```python
from build123d import *

# Parameters (mm, degrees)
F0_R     = 9
F1_DEPTH = 8
F2_R     = 3
F3_SIZE  = 7.99999
F4_SIZE2 = 7.7942286341
F4_SIZE  = 4.5


# Not quite as in the source:
# - a fillet or chamfer is up to 0.001 mm smaller than in the source, because OpenCascade refuses the exact size
# - ends of sketch curves that miss each other by under 0.0002 mm in the source are joined


with BuildPart() as f1:
    # F0 (on Front) → F1 (new body)
    with BuildSketch(Plane.XZ):
        with BuildLine():
            ThreePointArc((-43, -330.994167), (0, -287.994167), (43, -330.994167))
            ThreePointArc((43, -330.994167), (109.276026714, -321.904147751), (174.0000001055, -304.9941673237))
            Line((174.0000001055, -304.9941673237), (167.462801, -276.227606))
            Line((167.462801, -276.227606), (105.54156, -290.299203))
            ThreePointArc((105.54156, -290.299203), (85.7953886494, -277.8658315797), (98.2287608958, -258.1196605414))
            Line((98.2287608958, -258.1196605414), (160.150002, -244.048063))
            Line((160.150002, -244.048063), (101.992538, 11.87045))
            Line((101.992538, 11.87045), (133.663965, 45.228522))
            Line((133.663965, 45.228522), (88.338787, 88.261977))
            ThreePointArc((88.338787, 88.261977), (87.7337722092, 111.5886563014), (111.0604515643, 112.1936705411))
            Line((111.0604515643, 112.1936705411), (156.385629, 69.160216))
            Line((156.385629, 69.160216), (187.038105, 101.445071))
            Line((187.038105, 101.445071), (191.402576, 146.180902))
            Line((191.402576, 146.180902), (129.197911, 152.24965))
            ThreePointArc((129.197911, 152.24965), (114.3780295485, 170.2738304953), (132.4022099517, 185.0937125046))
            Line((132.4022099517, 185.0937125046), (194.606875, 179.024965))
            Line((194.606875, 179.024965), (198.96141, 223.658948))
            Line((198.96141, 223.658948), (169.162302, 256.167065))
            Line((169.162302, 256.167065), (123.090168, 213.934276))
            ThreePointArc((123.090168, 213.934276), (99.7776684169, 214.9478629238), (100.7912561729, 238.2603628114))
            Line((100.7912561729, 238.2603628114), (146.863389, 280.493152))
            Line((146.863389, 280.493152), (117.000674, 313.07066))
            Line((117.000674, 313.07066), (74.908309, 319.518852))
            Line((74.908309, 319.518852), (65.444247, 257.739555))
            ThreePointArc((65.444247, 257.739555), (46.6359995191, 243.928333625), (32.8247775616, 262.7365800672))
            Line((32.8247775616, 262.7365800672), (42.288841, 324.515877))
            Line((42.288841, 324.515877), (0, 330.994168))
            Line((0, 330.994168), (-42.288841, 324.515877))
            Line((-42.288841, 324.515877), (-32.824778, 262.73658))
            ThreePointArc((-32.824778, 262.73658), (-46.6360005191, 243.928333625), (-65.4442472887, 257.7395549558))
            Line((-65.4442472887, 257.7395549558), (-74.908309, 319.518852))
            Line((-74.908309, 319.518852), (-117.000674, 313.07066))
            Line((-117.000674, 313.07066), (-146.86339, 280.493152))
            Line((-146.86339, 280.493152), (-100.791256, 238.260363))
            ThreePointArc((-100.791256, 238.260363), (-99.7776686659, 214.9478626521), (-123.0901688686, 213.9342761433))
            Line((-123.0901688686, 213.9342761433), (-169.162302, 256.167065))
            Line((-169.162302, 256.167065), (-198.96141, 223.658948))
            Line((-198.96141, 223.658948), (-194.606875, 179.024965))
            Line((-194.606875, 179.024965), (-132.40221, 185.093713))
            ThreePointArc((-132.40221, 185.093713), (-114.3780295485, 170.2738304953), (-129.1979109611, 152.2496496015))
            Line((-129.1979109611, 152.2496496015), (-191.402576, 146.180902))
            Line((-191.402576, 146.180902), (-187.038105, 101.445071))
            Line((-187.038105, 101.445071), (-156.385629, 69.160216))
            Line((-156.385629, 69.160216), (-111.060452, 112.193671))
            ThreePointArc((-111.060452, 112.193671), (-87.7337732092, 111.5886563014), (-88.3387874357, 88.2619774589))
            Line((-88.3387874357, 88.2619774589), (-133.663965, 45.228522))
            Line((-133.663965, 45.228522), (-101.992538, 11.87045))
            Line((-101.992538, 11.87045), (-160.150002, -244.048063))
            Line((-160.150002, -244.048063), (-98.228761, -258.119661))
            ThreePointArc((-98.228761, -258.119661), (-85.7953886494, -277.8658315797), (-105.5415600551, -290.2992032425))
            Line((-105.5415600551, -290.2992032425), (-167.462801, -276.227606))
            Line((-167.462801, -276.227606), (-174, -304.994167))
            ThreePointArc((-174, -304.994167), (-109.276026714, -321.904147751), (-43, -330.994167))
        make_face()
        with BuildLine():
            Line((-69.5, -145.994167), (-43.5, -145.994167))
            Line((-43.5, -145.994167), (-43.5, -205.994167))
            Line((-43.5, -205.994167), (-79.5, -205.994167))
            Line((-79.5, -205.994167), (-79.5, -155.994167))
            ThreePointArc((-79.5, -155.994167), (-76.5710678119, -148.9230991881), (-69.5, -145.994167))
        make_face(mode=Mode.SUBTRACT)
        with BuildLine():
            Line((43.5, -205.994167), (43.5, -145.994167))
            Line((43.5, -145.994167), (69.5, -145.994167))
            ThreePointArc((69.5, -145.994167), (76.5710678119, -148.9230991881), (79.5, -155.994167))
            Line((79.5, -155.994167), (79.5, -205.994167))
            Line((79.5, -205.994167), (43.5, -205.994167))
        make_face(mode=Mode.SUBTRACT)
        with Locations((-62.5, 2.005833)):
            Circle(F0_R, mode=Mode.SUBTRACT)
        with Locations((-62.5, 52.005833)):
            Circle(F0_R, mode=Mode.SUBTRACT)
        with Locations((62.5, 2.005833)):
            Circle(F0_R, mode=Mode.SUBTRACT)
        with Locations((62.5, 52.005833)):
            Circle(F0_R, mode=Mode.SUBTRACT)
    extrude(amount=F1_DEPTH)

    # F2
    f2_edges = [f1.edges().sort_by_distance(p)[0] for p in [
        (-43.5, -4, -205.994167),
        (79.5, -4, -205.994167),
        (43.5, -4, -205.994167),
        (-79.5, -4, -205.994167),
        (-43.5, -4, -145.994167),
        (43.5, -4, -145.994167),
    ]]
    fillet(f2_edges, radius=F2_R)

    # F3 (size 8 in the source; OpenCascade refuses exactly that, so slightly less here)
    f3_edges = [f1.edges().sort_by_distance(p)[0] for p in [
        (-71.5, -8, 52.005833),
        (53.5, -8, 52.005833),
        (-71.5, -8, 2.005833),
        (53.5, -8, 2.005833),
        (-58, -8, -145.994167),
        (58, -8, -145.994167),
        (0, -8, -287.994167),
    ]]
    chamfer(f3_edges, length=F3_SIZE)

    # F4
    f4_edges = [f1.edges().sort_by_distance(p)[0] for p in [
        (-133.72304, -8, 90.676943),
        (-163.504543, -8, 182.059339),
        (-123.827323, -8, 259.376757),
        (-37.556809, -8, 293.626229),
        (70.176278, -8, 288.629204),
        (123.827323, -8, 259.376757),
        (163.504542, -8, 182.059339),
        (133.72304, -8, 90.676943),
        (129.189381, -8, -251.083862),
        (-129.189381, -8, -251.083862),
    ]]
    f4_side = f1.faces().sort_by_distance((0, -8, 8.818439))[0]
    chamfer(f4_edges, length=F4_SIZE, length2=F4_SIZE2, reference=f4_side)


solid = f1.part
```
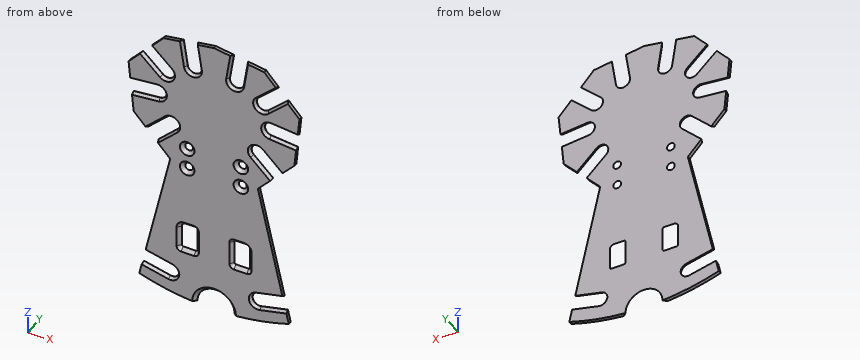
CAD build for the part. Positions are in the model's coordinates, mm. Coordinates: 2 decimals unless noted, no trailing zeros. Loops run counter-clockwise (first coordinate to the right, second up) from the corner with the lowest first, then second, coordinate; pieces in that order, holes last. Notation, with made-up numbers: (-18.75, -25) - (0.25, -25) arc R17 ccw to (0.25, -19) - close; hole circle Ø6 at (76, 87.25). An arc over 180 degrees is marked (long way). Use CSV: the item, a comma, the result in double quotes. Start each with the question number.
Q1. Drop flat-ended pins along their axis: P1, Ø3, axis at x = -61, z = -240.5, coming from the +Y side; P2, Ø11, axis at x = 62.5, z = 2.01, coming from the -Y side; P3, Ø3, axis at y = -4.5, z = -40, coming from the -X side; P4, Ø23.5, axis at x = -62.5, z = 2.01, coming from the -Y side. Give the stop position or say it passes through.
Q2. Cut at C-C, the plane z = -93. List the corners of the cut face in (x, y).
Q3. Cut at A-A, the plane z = 270. List the corners of the cut face in (x, y).
Q4. Probe probe 1 along Z at (x, y) = (168, -5); probe 2 along X at (y, z) = (-4, 82); probe 3 along X at (y, z) = (-2.25, 210.5). List the from-to ranges inside material, lowest first. Write a range as from..to.
Q5. Cut at B-B, the plane y = -2. State how many separate pieces and enclosed holes the cut face has, then the cut area to 3 significant figures.
Here are the results:
1,P1,"y = 0"
1,P2,"through"
1,P3,"x = -114.12"
1,P4,"y = -2.75"
2,outline,"(-125.82, -8) - (125.82, -8) - (125.82, 0) - (-125.82, 0) - close"
3,outline,"(-135.42, -0.21) - (-128.76, -8) - (-71.87, -8) - (-67.32, -0.21) - (-67.32, 0) - (-135.42, 0) - close; (-33.94, -0.21) - (-29.38, -8) - (29.38, -8) - (33.94, -0.21) - (33.94, 0) - (-33.94, 0) - close; (67.32, -0.21) - (71.87, -8) - (128.76, -8) - (135.42, -0.21) - (135.42, 0) - (67.32, 0) - close"
4,probe 1,"-306.91..-278.94, 81.39..145.68, 184.4..251.35"
4,probe 2,"-168.58..-146.04, -91.75..91.75, 146.04..168.58"
4,probe 3,"-197.68..-120.27, -103.62..103.62, 120.27..197.68"
5,separate pieces,"1"
5,enclosed holes,"6"
5,area,"161,000 mm2"
